Geometry check sheet. Reference: the model listing, model coordinates, mm. A direction names the side the tool comes from. Round coordinates to 2 decimals unless told otherwise and drop trailing zeros.
Item 1: Access from +Z, -Z, +X, -X, +Y, -Y to the whole of each face (thin tool, end or side, straight path). Record for faces 1 (the face through (22.688, -12.874, -11.374)), 2 (the face through (14.983, -12.016, 17.902)), 3 (the face through (-16, 0, 25)).
Item 2: Cross-section at A-A (y = -9). State how many separate pieces and enclosed holes the cut face has, then the cut area to 3 significant figures.
Item 3: Scan lines: probe 1 along Z at (x, y) = (-25, -11.5); probe 2 along Z at (x, y) = (-23, -13); probe 3 along X at (y, z) = (-12.5, 3). Record each from-to range of solid material in increasing order.
Item 4: Draft check along Z on faces 4 (the face through (13.772, 13.295, 9.957)), 5 (the face through (-35, 0, 0)), 6 (the face through (-32, -23, 5)), 7 (the face through (-16, 0, -25)). Enter one of: pulls with the +Z half, pulls with the -Z half, needs draft (parallel to the pull), parting line crosses it, or undercut.
Item 5: Depth check by flat-ended pin: P1, Ø2.5, axis at x = -13.44, y = 13.44, coming from the +Z side; P2, Ø7, axis at x = -26, z = -18.5, coming from the -Y side; P3, Ø12.5, axis at x = 25, z = -15, coming from the -Y side. Enter the tip coordinate at first touch or a pass-through.
from build123d import *

# Parameters (mm, degrees)
ESQUISSE1_W                                        = 70
ESQUISSE1_H                                        = 50
BOSS_EXTRU_1_DEPTH                                 = 48
D_GAGEMENT_M251_D                                  = 28.4
DIAM_TRE_DU_PER_AGE_4_2_4_2_1_D                    = 4.2
DIAM_TRE_DU_PER_AGE_4_2_4_2_1_DEPTH                = 14
DIAM_TRE_DU_PER_AGE_4_2_4_2_1_TIP                  = 1.2618073
CHAMBRAGE_POUR_VIS_T_TE_HEXAGONALE_M81_D           = 8.6
CHAMBRAGE_POUR_VIS_T_TE_HEXAGONALE_M81_DEPTH       = 20
CHAMBRAGE_POUR_VIS_T_TE_HEXAGONALE_M81_CBORE_D     = 14
CHAMBRAGE_POUR_VIS_T_TE_HEXAGONALE_M81_CBORE_DEPTH = 2
CHAMBRAGE_POUR_VIS_T_TE_HEXAGONALE_M81_TIP         = 2.583700662
CHANFREIN1_SIZE                                    = 0.5
CHANFREIN2_SIZE                                    = 1


with BuildPart() as part:
    # Esquisse1 → Boss.-Extru.1 (new body)
    with BuildSketch(Plane.XZ.offset(24)):
        Rectangle(ESQUISSE1_W, ESQUISSE1_H)
    extrude(amount=-BOSS_EXTRU_1_DEPTH)

    # Dégagement M251 (through all)
    with Locations(Plane(origin=(0, 0, -25), x_dir=(-1, 0, 0), z_dir=(0, 0, -1))):
        with Locations((0, 0)):
            Hole(D_GAGEMENT_M251_D / 2)

    # Diamètre du perçage Ø4.2 (4.2)1
    with Locations(Plane.XY.offset(25)):
        with Locations((13.435028843, -13.435028843), (13.435028843, 13.435028843), (19, 0), (-13.435028843, 13.435028843), (-13.435028843, -13.435028843), (-19, 0)):
            Hole(DIAM_TRE_DU_PER_AGE_4_2_4_2_1_D / 2, depth=DIAM_TRE_DU_PER_AGE_4_2_4_2_1_DEPTH)
            with Locations((0, 0, -(DIAM_TRE_DU_PER_AGE_4_2_4_2_1_DEPTH + DIAM_TRE_DU_PER_AGE_4_2_4_2_1_TIP / 2))):  # 118° drill point
                Cone(0, DIAM_TRE_DU_PER_AGE_4_2_4_2_1_D / 2, DIAM_TRE_DU_PER_AGE_4_2_4_2_1_TIP, mode=Mode.SUBTRACT)

    # Chambrage pour vis à tête hexagonale M81
    with Locations(Plane.XZ.offset(24)):
        with Locations((25, 5), (25, -15), (-25, 5), (-25, -15)):
            CounterBoreHole(CHAMBRAGE_POUR_VIS_T_TE_HEXAGONALE_M81_D / 2, CHAMBRAGE_POUR_VIS_T_TE_HEXAGONALE_M81_CBORE_D / 2, CHAMBRAGE_POUR_VIS_T_TE_HEXAGONALE_M81_CBORE_DEPTH, depth=CHAMBRAGE_POUR_VIS_T_TE_HEXAGONALE_M81_DEPTH)
            with Locations((0, 0, -(CHAMBRAGE_POUR_VIS_T_TE_HEXAGONALE_M81_DEPTH + CHAMBRAGE_POUR_VIS_T_TE_HEXAGONALE_M81_TIP / 2))):  # 118° drill point
                Cone(0, CHAMBRAGE_POUR_VIS_T_TE_HEXAGONALE_M81_D / 2, CHAMBRAGE_POUR_VIS_T_TE_HEXAGONALE_M81_TIP, mode=Mode.SUBTRACT)

    # Chanfrein1
    chanfrein1_edges = [part.edges().sort_by_distance(p)[0] for p in [
        (-32, -24, -15),
        (-32, -24, 5),
        (18, -24, -15),
        (18, -24, 5),
    ]]
    chamfer(chanfrein1_edges, length=CHANFREIN1_SIZE)

    # Chanfrein2
    chanfrein2_edges = [part.edges().sort_by_distance(p)[0] for p in [
        (35, 24, 0),
        (0, 24, 25),
        (-14.2, 0, -25),
        (-14.2, 0, 25),
        (-35, 24, 0),
        (0, -24, 25),
        (35, -24, 0),
        (0, -24, -25),
        (-35, -24, 0),
        (0, 24, -25),
        (-35, 0, 25),
        (35, 0, 25),
        (35, 0, -25),
        (-35, 0, -25),
    ]]
    chamfer(chanfrein2_edges, length=CHANFREIN2_SIZE)


solid = part.part
Resolved:
1. face 1: -Y
1. face 2: +Z
1. face 3: +Z, +X, -X, +Y, -Y
2. separate pieces: 2
2. enclosed holes: 4
2. area: 2,160 mm2
3. probe 1: z = -25 to -19.3, -10.7 to 0.7, 9.3 to 25
3. probe 2: z = -25 to -18.81, -11.19 to 1.19, 8.81 to 25
3. probe 3: x = -35 to -28.81, -21.19 to -6.74, 6.74 to 21.19, 28.81 to 35
4. face 4: pulls with the +Z half
4. face 5: needs draft
4. face 6: undercut
4. face 7: pulls with the -Z half
5. P1: stops at z = 10.49
5. P2: stops at y = -23.64
5. P3: stops at y = -22
